Autodesk Inventor part; units mm, degrees
ref_plane "YZ Plane" through (0, 0, 0) normal (1, 0, 0) x (0, 1, 0)
ref_plane "XZ Plane" through (0, 0, 0) normal (0, 1, 0) x (-1, 0, 0)
ref_plane "XY Plane" through (0, 0, 0) normal (0, 0, 1) x (1, 0, 0)
sketch "Sketch1" plane through (0, 0, 0) normal (0, 0, 1) x (1, 0, 0)
  circle A0 centre (0, 0) radius 16.764
  circle A1 centre (0, 0) radius 23.114
  line L0 (23.114, 0) -> (23.114, -73.914)
  line L1 (23.114, -73.914) -> (-23.114, -73.914)
  line L2 (-23.114, -73.914) -> (-23.114, 0)
  line L3 (23.114, -23.114) -> (0, -23.114)
  line L4 (-23.114, -23.114) -> (0, -23.114)
  dimension "d0" = 33.528
  dimension "d1" = 6.35
  dimension "d23" = 50.8
extrude "Extrusion2" add sketch "Sketch1" along normal blind 25.4
sketch "Sketch3" plane through (0, 0, 25.4) normal (0, 0, 1) x (1, 0, 0)
  line L0 (-23.114, 0) -> (-23.114, -73.914)
  line L1 (23.114, -73.914) -> (23.114, 0)
  line L2 (-23.114, -73.914) -> (23.114, -73.914)
  line L3 (23.114, -73.914) -> (23.114, -23.114)
  line L4 (23.114, -23.114) -> (-23.114, -23.114)
  line L5 (-23.114, -23.114) -> (-23.114, -73.914)
  arc A0 (23.114, 0) -> (-23.114, 0) centre (0, 0) ccw
  circle A1 centre (0, 0) radius 23.114
  line L6 (-23.114, -73.914) -> (23.114, -73.914)
  line L7 (0, -23.114) -> (0, -73.914)
  point P0 (0, -54.864)
  dimension "d24" = 19.05
hole "Hole1" at (0, -54.864, 25.4) direction (0, 0, -1) diameter 19.8374 end through all
sketch "Sketch6" plane through (-23.114, -73.914, 0) normal (0, -1, 0) x (1, 0, 0)
  line L0 (46.228, 0) -> (46.228, 25.4)
  line L1 (0, 0) -> (0, 25.4)
  line L2 (46.228, 8.255) -> (0, 8.255)
  line L3 (0, 8.255) -> (0, 17.145)
  line L4 (0, 17.145) -> (46.228, 17.145)
  line L5 (46.228, 17.145) -> (46.228, 8.255)
  line L6 (46.228, 25.4) -> (0, 25.4)
  line L7 (46.228, 0) -> (0, 0)
  point P0 (23.114, 0)
  dimension "d18" = 8.89
  dimension "d19" = 8.255
extrude "Extrusion3" cut sketch "Sketch6" against normal blind 50.8 contours L2 L1 L4 L0
sketch "Sketch7" plane through (0, 0, 25.4) normal (0, 0, 1) x (1, 0, 0)
  circle A0 centre (0, -54.864) radius 9.9187
  circle A1 centre (0, 0) radius 16.764
  dimension "d25" = 54.864
equation "\"d23\" = MountingArmLength"
equation "\"d19\" = ArmWidth"
equation "\"d20\" = MountingArmLength"
equation "\"ArmWidth\" = -0.5 * d18 + 0.5 * d7"
equation "\"ArmOffsetDist\" = d25"
properties part number "FrameMountingBracket"
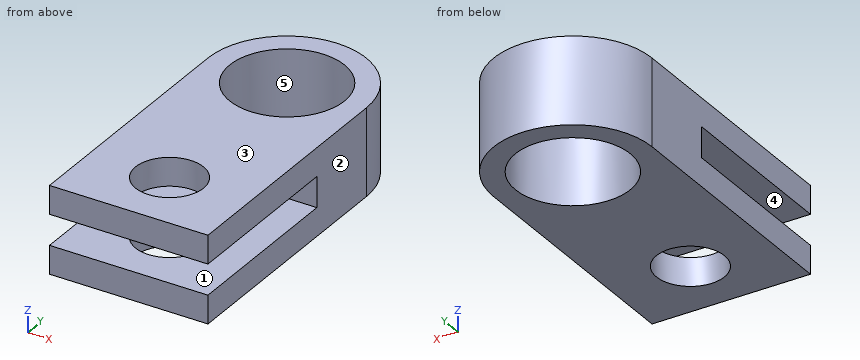
Design review of the part built by this model. Coordinates are the model's own, in mm. Face numbers are marked on the shaded views. A direction names the side the tool comes from. Coordinates: 2 decimals unless noted, no trailing zeros. Write each loop counter-clockwise with the first axis right and the second up, starting at its lowest first coordinate (ties: lowest second). Pieces come first, ordered by that corner, then holes. Notation, with made-up numbers: (6, 82) - (47, 82) arc R29 ccw to (47, 103) - close; hole circle Ø1 at (23.5, 18). An arc over 180 degrees is marked (long way). One line per item, written item: value.
1) Mouldability with a two-part tool opening along Z and no side actions: class the marked faces 1, 2 and 3 as +Z half, -Z half, draft (parallel to the pull), parting line (faces both ways), or undercut.
Answer sheet:
face 1: undercut
face 2: draft
face 3: +Z half
2) Add section A-A (x = 0). State the section outline as (y, z) points (3 decimals).
Answer sheet:
outline: (-73.914, 0) - (-64.783, 0) - (-64.783, 8.255) - (-73.914, 8.255) - close; (-73.914, 17.145) - (-64.783, 17.145) - (-64.783, 25.4) - (-73.914, 25.4) - close; (-44.945, 0) - (-16.764, 0) - (-16.764, 25.4) - (-44.945, 25.4) - (-44.945, 17.145) - (-23.114, 17.145) - (-23.114, 8.255) - (-44.945, 8.255) - close; (16.764, 0) - (23.114, 0) - (23.114, 25.4) - (16.764, 25.4) - close
3) To check wall thickness, follow probe 1 along Y at (x, z) = (0, 22); probe 2 along Z at (x, y) = (-10.5, -59) (3 decimals); probe 3 along Y at (x, z) = (-8, 3.25). State the ranges of each line that lie inside material, in increasing order.
Answer sheet:
probe 1: y = -73.91 to -64.78, -44.95 to -16.76, 16.76 to 23.11
probe 2: z = 0 to 8.255, 17.145 to 25.4
probe 3: y = -73.91 to -60.73, -49 to -14.73, 14.73 to 21.69
4) Add section C-C (z = 12.5). State the section outline as (x, y) points, plus the area to 3 significant figures.
Answer sheet:
outline: (-23.11, -23.11) - (23.11, -23.11) - (23.11, 0) arc R23.11 ccw to (-23.11, 0) - close; hole circle Ø33.53 at (0, 0)
area: 1,020 mm2
5) Insertion check: pin 1 (1.5 mm diameter, centred on x = -9.5, z = 17, fed in from +Y); pin 2 (10 mm diameter, centred on y = 1.5, z = 21.5, fed in from +X); pin 3 (12 mm diameter, centred on x = 0, y = -54.864, fed in from +Z); pin 4 (6 mm diameter, centred on y = 10.5, z = 13.5, fed in from -X). Each pin has a flat end and moves straight along its axis. Give the tip position at first contact, or say it passes through.
Answer sheet:
pin 1: stops at y = 21.39
pin 2: stops at x = 23.11
pin 3: passes through
pin 4: stops at x = -21.86
6) Add section D-D (z = 18.75). State the section outline as (x, y) points, plus the area to 3 significant figures.
Answer sheet:
outline: (-23.11, -73.91) - (23.11, -73.91) - (23.11, 0) arc R23.11 ccw to (-23.11, 0) - close; hole circle Ø33.53 at (0, 0); hole circle Ø19.84 at (0, -54.86)
area: 3,060 mm2
7) For the marked faces 4 and 5, list the 3-axis set-ups (+Z, -Z, +X, -X, +Y, -Y) from which the entire face can be reached by the end or side of a thin tool; tool diameter is ignored.
Answer sheet:
face 4: +X, -X, -Y
face 5: +Z, -Z
8) Add section B-B (y = -27). State the section outline as (x, z) points (3 decimals), plus the area to 3 significant figures.
Answer sheet:
outline: (-23.114, 0) - (23.114, 0) - (23.114, 8.255) - (-23.114, 8.255) - close; (-23.114, 17.145) - (23.114, 17.145) - (23.114, 25.4) - (-23.114, 25.4) - close
area: 763 mm2
